Could you check a few things on this model? Use its own coordinates, in mm. Face numbers are marked on the shaded views. Coordinates: 2 decimals unless noted, no trailing zeros. Write each loop counter-clockwise with the first axis right and the second up, starting at its lowest first coordinate (ties: lowest second). Pieces come first, ordered by that corner, then holes. Notation, with made-up numbers: (36, -5) - (40, -5) arc R25 ccw to (40, 21) - close; hole circle Ø4 at (-19, 87.5). An arc over 180 degrees is marked (long way). Write item = value, one per line. Start each with the question number.
```python
from build123d import *

# Parameters (mm, degrees)
F2_R     = 18.5
F2_R_2   = 17
F2_R_3   = 5.15
F2_R_4   = 0.5
F3_DEPTH = 0.4
F4_DEPTH = 1.5
F5_DEPTH = 12


with BuildPart() as f3:
    # F2 (on Top) → F3 (new body)
    with BuildSketch(Plane.XY):
        Circle(F2_R)
        Circle(F2_R_2, mode=Mode.SUBTRACT)
        Circle(F2_R_2)
        with Locations((0, -11)):
            Circle(F2_R_3, mode=Mode.SUBTRACT)
        with Locations((-11.2583302492, 6.5)):
            Circle(F2_R_4, mode=Mode.SUBTRACT)
        Circle(F2_R_3, mode=Mode.SUBTRACT)
        with Locations((11.2583302492, 6.5)):
            Circle(F2_R_4, mode=Mode.SUBTRACT)
        with Locations((0, 11)):
            Circle(F2_R_3, mode=Mode.SUBTRACT)
        with Locations((0, -11)):
            Circle(F2_R_3)
        with Locations((0, -13)):
            Circle(F2_R_4, mode=Mode.SUBTRACT)
        Circle(F2_R_3)
        with Locations((0, 11)):
            Circle(F2_R_3)
    extrude(amount=-F3_DEPTH)

    # F2 (on Top) → F4 (join)
    with BuildSketch(Plane.XY):
        Circle(F2_R_2)
        with Locations((0, -11)):
            Circle(F2_R_3, mode=Mode.SUBTRACT)
        with Locations((-11.2583302492, 6.5)):
            Circle(F2_R_4, mode=Mode.SUBTRACT)
        Circle(F2_R_3, mode=Mode.SUBTRACT)
        with Locations((11.2583302492, 6.5)):
            Circle(F2_R_4, mode=Mode.SUBTRACT)
        with Locations((0, 11)):
            Circle(F2_R_3, mode=Mode.SUBTRACT)
        with Locations((0, 11)):
            Circle(F2_R_3)
        with Locations((0, -11)):
            Circle(F2_R_3)
        with Locations((0, -13)):
            Circle(F2_R_4, mode=Mode.SUBTRACT)
    extrude(amount=F4_DEPTH)

    # F2 (on Top) → F5 (join)
    with BuildSketch(Plane.XY):
        Circle(F2_R)
        Circle(F2_R_2, mode=Mode.SUBTRACT)
    extrude(amount=F5_DEPTH)


solid = f3.part
```
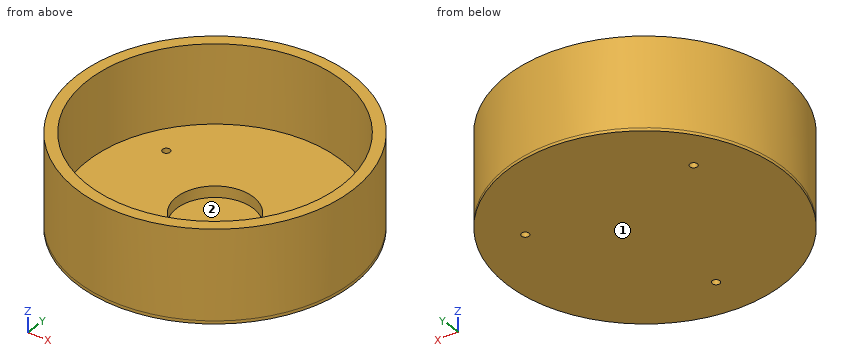
1) Suppose I cut it at B-B on y = 6.5. Please give me the cut outline in (x, z), plus the area to 3 significant figures.
2) For P1, Ø4, axis at x = -6, z = 7.5, coming from the +Y side; P2, Ø1, axis at y = -4.5, z = 3, coming from the -X side; P3, Ø3, axis at y = 13, z = 8, coming from the +X side, each with a flat end and sliding along its axis, tell me the tip position at first contact or that it passes through.
3) Suppose I cut it at A-A on x = 0. Please give me the cut outline in (y, z).
4) Suppose I cut it at C-C on y = -13. Please give me the cut outline in (x, z), plus the area to 3 significant figures.
5) Suppose I cut it at D-D on z = 1. Please give me the cut outline in (x, y), plus the area to 3 significant figures.
6) If I drill on probe 1 along Y at (x, z) = (0, 0.85); probe 2 along Z at (x, y) = (4, 5); probe 3 along Y at (x, z) = (-10, 6.75), over which ranges is the centre line in solid material (lowest first)? Write a range as [from, to].
7) Thinking about a two-plate mould opening in Y: for the marked faces 1 and 2, which applies, +Y half, -Y half, draft (parallel to the pull), parting line (faces both ways), or undercut?
Reply:
q1.outline = (-17.32, -0.4) - (-11.76, -0.4) - (-11.76, 1.5) - (-15.71, 1.5) - (-15.71, 12) - (-17.32, 12) - close; (-10.76, -0.4) - (10.76, -0.4) - (10.76, 1.5) - (-10.76, 1.5) - close; (11.76, -0.4) - (17.32, -0.4) - (17.32, 12) - (15.71, 12) - (15.71, 1.5) - (11.76, 1.5) - close
q1.area = 95.9 mm^2
q2.P1 = 18.06
q2.P2 = -18.06
q2.P3 = 14.49
q3.outline = (-18.5, -0.4) - (-13.5, -0.4) - (-13.5, 1.5) - (-17, 1.5) - (-17, 12) - (-18.5, 12) - close; (-12.5, -0.4) - (18.5, -0.4) - (18.5, 12) - (17, 12) - (17, 1.5) - (5.15, 1.5) - (5.15, 0) - (-5.15, 0) - (-5.15, 1.5) - (-12.5, 1.5) - close
q4.outline = (-13.16, -0.4) - (-0.5, -0.4) - (-0.5, 1.5) - (-10.95, 1.5) - (-10.95, 12) - (-13.16, 12) - close; (0.5, -0.4) - (13.16, -0.4) - (13.16, 12) - (10.95, 12) - (10.95, 1.5) - (0.5, 1.5) - close
q4.area = 94.5 mm^2
q5.outline = circle Ø37 at (0, 0); hole circle Ø1 at (-11.26, 6.5); hole circle Ø10.3 at (0, 0); hole circle Ø1 at (0, -13); hole circle Ø1 at (11.26, 6.5)
q5.area = 990 mm^2
q6.probe_1 = [-18.5, -13.5], [-12.5, -5.15], [5.15, 18.5]
q6.probe_2 = [-0.4, 1.5]
q6.probe_3 = [-15.56, -13.75], [13.75, 15.56]
q7.face_1 = draft
q7.face_2 = undercut
